Autodesk Inventor part; units mm, degrees
ref_plane "XZ Plane" through (0, 0, 0) normal (0, 1, 0) x (-1, 0, 0)
ref_plane "XY Plane" through (0, 0, 0) normal (0, 0, 1) x (1, 0, 0)
sketch "Sketch1" plane through (0, 0, 0) normal (0, 0, 1) x (1, 0, 0)
  line L0 (-25.4, -25.4) -> (25.4, -25.4)
  line L1 (25.4, -25.4) -> (25.4, 25.4)
  line L2 (25.4, 25.4) -> (-25.4, 25.4)
  line L3 (-25.4, 25.4) -> (-25.4, -25.4)
  line L4 (-25.4, -25.4) -> (25.4, 25.4) construction
  line L5 (25.4, -25.4) -> (-25.4, 25.4) construction
  line L6 (-22.225, -22.225) -> (22.225, -22.225)
  line L7 (22.225, -22.225) -> (22.225, 22.225)
  line L8 (22.225, 22.225) -> (-22.225, 22.225)
  line L9 (-22.225, 22.225) -> (-22.225, -22.225)
  line L10 (-22.225, -22.225) -> (22.225, 22.225) construction
  line L11 (22.225, -22.225) -> (-22.225, 22.225) construction
  point P0 (0, 0)
  dimension "d0" = 50.8
  dimension "d1" = 3.175
extrude "Extrusion1" add sketch "Sketch1" against normal blind 800.1
sketch "Sketch2" plane through (25.4, -25.4, 0) normal (1, 0, 0) x (0, 0, -1)
  circle A0 centre (76.2, 25.4) radius 12.7
  line L0 (0, 0) -> (0, 50.8)
  point P0 (0, 25.4)
  dimension "d4" = 25.4
  dimension "d7" = 76.2
extrude "Extrusion2" cut sketch "Sketch2" against normal through all
properties part number "2inSquareArmTube"
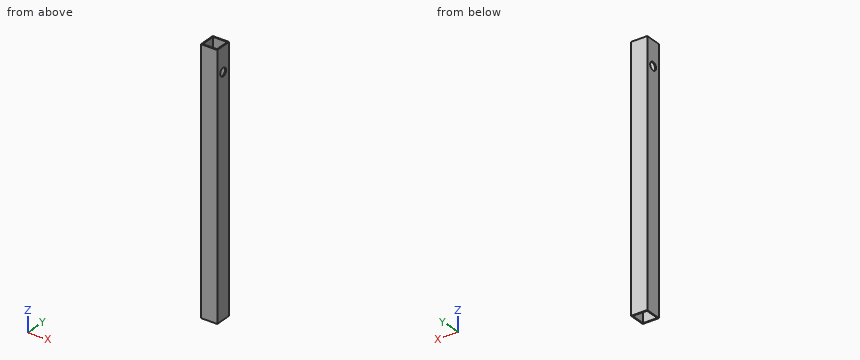
The listing builds one solid part. Answer for the finished solid, in the listing's coordinates (mm). Coordinates: 2 decimals unless noted, no trailing zeros. Order: outer loops, then holes, each group sorted by start corner. A loop starts at its lowest first (then second) coordinate and runs counter-clockwise, first axis right, second up.
Q1. A cutting plane is placed at D-D, the plane y = 0. Write down the section's boundary in (x, z) (3 decimals).
Q2. Consider line 1 (X direction, y = 5, z = -271.5) (3 decimals); line 2 (Y direction, x = 23, z = -76). Determine where each line is inside the solid, lowest interval first.
Q3. A cutting plane is placed at B-B, the plane z = -76.2. Write down the section's boundary in (x, y) (3 decimals), and give its area (3 significant figures).
Q4. A cutting plane is placed at A-A, the plane x = -12.5. Write down the section's boundary in (y, z) (3 decimals), and give its area (3 significant figures).
Q5. A cutting plane is placed at C-C, the plane z = -396. Write down the section's boundary in (x, y) (3 decimals), and give its area (3 significant figures).
Answers follow:
1. outline: (-25.4, -800.1) - (-22.225, -800.1) - (-22.225, -88.9) - (-25.4, -88.9) - close; (-25.4, -63.5) - (-22.225, -63.5) - (-22.225, 0) - (-25.4, 0) - close; (22.225, -800.1) - (25.4, -800.1) - (25.4, -88.9) - (22.225, -88.9) - close; (22.225, -63.5) - (25.4, -63.5) - (25.4, 0) - (22.225, 0) - close
2. line 1: x = -25.4 to -22.225, 22.225 to 25.4
2. line 2: y = -25.4 to -12.7, 12.7 to 25.4
3. outline: (-25.4, -25.4) - (25.4, -25.4) - (25.4, -12.7) - (22.225, -12.7) - (22.225, -22.225) - (-22.225, -22.225) - (-22.225, -12.7) - (-25.4, -12.7) - close; (-25.4, 12.7) - (-22.225, 12.7) - (-22.225, 22.225) - (22.225, 22.225) - (22.225, 12.7) - (25.4, 12.7) - (25.4, 25.4) - (-25.4, 25.4) - close
3. area: 444 mm2
4. outline: (-25.4, -800.1) - (-22.225, -800.1) - (-22.225, 0) - (-25.4, 0) - close; (22.225, -800.1) - (25.4, -800.1) - (25.4, 0) - (22.225, 0) - close
4. area: 5,080 mm2
5. outline: (-25.4, -25.4) - (25.4, -25.4) - (25.4, 25.4) - (-25.4, 25.4) - close; hole (-22.225, -22.225) - (22.225, -22.225) - (22.225, 22.225) - (-22.225, 22.225) - close
5. area: 605 mm2
